Read the model definition and answer for the solid it produces. Units are mm, in the model's axes. A direction names the side the tool comes from. Round coordinates to 2 decimals unless told otherwise and drop trailing zeros. Write each loop counter-clockwise with the first axis right and the second up, starting at its lowest first coordinate (ties: lowest second). Pieces come first, ordered by that corner, then holes. Notation, with made-up numbers: (40, -35) -> (96, -35) arc R18 cw to (96, -26) -> close; hole circle Ø8 at (29.5, 85.25). An arc over 180 degrees is marked (long way). Return JSON: item names as keys, results as strings.
from build123d import *

# Parameters (mm, degrees)
F0_R     = 10.16
F1_DEPTH = 50.8
F0_W     = 50.8
F0_H     = 44.45
F2_DEPTH = 2.54
F5_DEPTH = 1.27
F3_W     = 50.8
F3_H     = 6.35
F6_DEPTH = 1.27
F7_R     = 4.2926
F8_DEPTH = 6.351


with BuildPart() as f1:
    # F0 (on Front) → F1 (new body)
    with BuildSketch(Plane.XZ):
        Polygon((19.978336, 18.750969), (-56.221664, 18.750969), (-56.221664, 12.400969), (-5.421664, 12.400969), (-5.421664, -32.049031), (19.978336, -32.049031), align=None)
        with Locations((7.978835, -19.349031)):
            Circle(F0_R, mode=Mode.SUBTRACT)
        with Locations((7.978835, 6.050969)):
            Circle(F0_R, mode=Mode.SUBTRACT)
    extrude(amount=F1_DEPTH)

    # F0 (on Front) → F2 (join)
    with BuildSketch(Plane.XZ):
        with Locations((-30.821664, -9.824031)):
            Rectangle(F0_W, F0_H)
        with Locations((7.978835, -19.349031)):
            Circle(F0_R)
        with Locations((7.978835, 6.050969)):
            Circle(F0_R)
    extrude(amount=F2_DEPTH)

    # F4 (on face) → F5 (join)
    with BuildSketch(Plane(origin=(-56.221664, 0, 0), x_dir=(0, -1, 0), z_dir=(-1, 0, 0))):
        Polygon((8.878232, 12.400969), (2.54, 12.400969), (2.54, -32.049031), (8.878232, -32.435447), align=None)
    extrude(amount=-F5_DEPTH)

    # F3 (on face) → F6 (join)
    with BuildSketch(Plane(origin=(0, 0, -32.049031), x_dir=(1, 0, 0), z_dir=(0, 0, -1))):
        with Locations((-30.821664, 5.715)):
            Rectangle(F3_W, F3_H)
    extrude(amount=-F6_DEPTH)

    # F7 (on face) → F8 (cut, through all)
    with BuildSketch(Plane(origin=(0, 0, 12.400969), x_dir=(1, 0, 0), z_dir=(0, 0, -1))):
        with Locations((-44.832879, 35.587724)):
            Circle(F7_R)
        with Locations((-23.242238, 17.584552)):
            Circle(F7_R)
    extrude(amount=-F8_DEPTH, mode=Mode.SUBTRACT)


solid = f1.part
Item 1: Section B-B (y = -34) is taken. Give the vertices of the cut face in (x, z).
Worked answers:
{"outline": "(-56.22, 12.4) -> (-48.82, 12.4) -> (-48.82, 18.75) -> (-56.22, 18.75) -> close; (-40.84, 12.4) -> (-5.42, 12.4) -> (-5.42, -32.05) -> (19.98, -32.05) -> (19.98, 18.75) -> (-40.84, 18.75) -> close; hole circle Ø20.32 at (7.98, -19.35); hole circle Ø20.32 at (7.98, 6.05)"}
Item 2: Section A-A (x = -43.5) is taken. Give the vertices of the cut face in (y, z), then the cut area to 3 significant figures.
Worked answers:
{"outline": "(-50.8, 12.4) -> (-39.67, 12.4) -> (-39.67, 18.75) -> (-50.8, 18.75) -> close; (-31.51, 12.4) -> (-2.54, 12.4) -> (-2.54, -30.78) -> (-8.89, -30.78) -> (-8.89, -32.05) -> (0, -32.05) -> (0, 18.75) -> (-31.51, 18.75) -> close", "area": "392 mm2"}
Item 3: For a pull along Z with two mould halves and no side action, classify faces 1 (the flat face through (-2, -19, -32.049)), 2 (the flat face through (19.978, -25, -7)), 3 (the flat face through (-54.952, -6, -9)) as released by +Z, released by -Z, zero draft, split by the parting line, or undercut.
Worked answers:
{"face 1": "released by -Z", "face 2": "zero draft", "face 3": "undercut"}
Item 4: Flat-ended cylindrical pins translate along their axes: pin 1 (1 mm diameter, centred on x = -43, z = -31.5, fed in from -Y); pin 2 (7 mm diameter, centred on x = -44.83, y = -35.59, fed in from +Z); pin 3 (1 mm diameter, centred on x = 10, z = 3.5, fed in from -Y); pin 4 (4 mm diameter, centred on x = -18, y = -22.5, fed in from -Z). Find the tip coordinate at first contact, or state that the pin passes through.
Worked answers:
{"pin 1": "stops at y = -8.89", "pin 2": "passes through", "pin 3": "stops at y = -2.54", "pin 4": "stops at z = 12.4"}
Item 5: Section D-D (z = -3) is taken. Give the vertices of the cut face in (x, y).
Worked answers:
{"outline": "(-56.22, -8.88) -> (-54.95, -8.88) -> (-54.95, -2.54) -> (-5.42, -2.54) -> (-5.42, -50.8) -> (3.36, -50.8) -> (3.36, -2.54) -> (12.59, -2.54) -> (12.59, -50.8) -> (19.98, -50.8) -> (19.98, 0) -> (-56.22, 0) -> close"}
Item 6: Section C-C (y = -41.5) is taken. Give the vertices of the cut face in (x, z), then the cut area to 3 significant figures.
Worked answers:
{"outline": "(-56.22, 12.4) -> (-5.42, 12.4) -> (-5.42, -32.05) -> (19.98, -32.05) -> (19.98, 18.75) -> (-56.22, 18.75) -> close; hole circle Ø20.32 at (7.98, -19.35); hole circle Ø20.32 at (7.98, 6.05)", "area": "964 mm2"}
Item 7: Straight lines are drawn through the part: L1, parallel to X at y = -7.5, z = -20.5; L2, parallel to Z at x = -0.5, y = -26.5; L3, parallel to X at y = -7, z = 0.5. For each, find the intervals that lie inside material, in ascending order. Write a range as [from, to].
Worked answers:
{"L1": "x = [-56.22, -54.95], [-5.42, -2.12], [18.07, 19.98]", "L2": "z = [-32.05, -24.95], [-13.75, 0.45], [11.65, 18.75]", "L3": "x = [-56.22, -54.95], [-5.42, -0.53], [16.49, 19.98]"}
Item 8: A tool of negligible diameter and unlimited length cuts with its end or side. For faces 4 (the flat face through (8, -2.54, 6)), 5 (the flat face through (-19, 0, -6)), from which of +Z, -Z, +X, -X, +Y, -Y can it reach the whole face along a straight path? Write none if from no direction.
Worked answers:
{"face 4": "-Y", "face 5": "+Z, -Z, +X, -X, +Y"}
